from build123d import *

# Parameters (mm, degrees)
SKETCH_W        = 65
SKETCH_H        = 65
PAD_DEPTH       = 16
SKETCH001_W     = 45
SKETCH001_H     = 45
POCKET_DEPTH    = 6
CHAMFER_SIZE    = 13
CHAMFER001_SIZE = 6
CHAMFER002_SIZE = 3


with BuildPart() as part:
    # Sketch → Pad (new body)
    with BuildSketch(Plane.XY):
        with Locations((32.5, 32.5)):
            Rectangle(SKETCH_W, SKETCH_H)
    extrude(amount=PAD_DEPTH)

    # Sketch001 (on Face6 of Pad) → Pocket (cut)
    with BuildSketch(Plane.XY.offset(16)):
        with Locations((32.5, 32.5)):
            Rectangle(SKETCH001_W, SKETCH001_H)
    extrude(amount=-POCKET_DEPTH, mode=Mode.SUBTRACT)

    # Chamfer
    chamfer_edges = [part.edges().sort_by_distance(p)[0] for p in [
        (0, 0, 8),
        (65, 0, 8),
        (65, 65, 8),
        (0, 65, 8),
    ]]
    chamfer(chamfer_edges, length=CHAMFER_SIZE)

    # Chamfer001
    chamfer001_edges = [part.edges().sort_by_distance(p)[0] for p in [
        (32.5, 0, 16),
        (65, 32.5, 16),
        (32.5, 65, 16),
        (0, 32.5, 16),
    ]]
    chamfer(chamfer001_edges, length=CHAMFER001_SIZE)

    # Chamfer002
    chamfer002_edges = [part.edges().sort_by_distance(p)[0] for p in [
        (32.5, 0, 10),
        (65, 32.5, 10),
        (32.5, 65, 10),
        (0, 32.5, 10),
    ]]
    chamfer(chamfer002_edges, length=CHAMFER002_SIZE)


solid = part.part
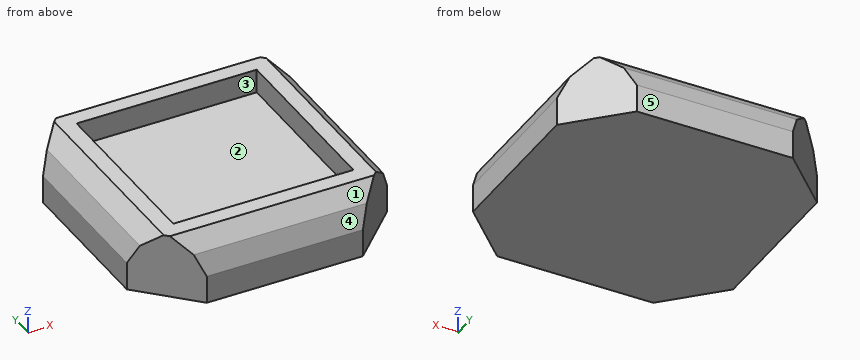
Verification items for the finished model (mm, model axes). Face numbers are marked on the shaded views. A direction names the side the tool comes from. Coordinates: 2 decimals unless noted, no trailing zeros. Order: outer loops, then holes, each group sorted by start corner. A loop starts at its lowest first (then second) coordinate and runs counter-clockwise, first axis right, second up. Notation, with made-up numbers: M 31.25,27 L 37.25,27 A15 cw 37.25,43 Z; hole C -4.75,-38.75 d3. An arc over 180 degrees is marked long. One line per item, written item: value. Start each with the question number.
Item 1: Depth check by flat-ended pin: P1, Ø13.5, axis at x = 34, y = 23.5, coming from the +Z side; P2, Ø1.8, axis at y = 34.5, z = 13, coming from the -X side; P3, Ø4, axis at x = 9, z = 12.5, coming from the +Y side. Enter the tip coordinate at first touch or a pass-through.
Item 2: Sectioned sample at A-A on z = 13.25. Record the cut outline in (x, y), then the cut area to 3 significant figures.
Item 3: Thickness scan on probe 1 along Y at (x, z) = (48, 14.75); probe 2 along Z at (x, y) = (51.5, 29); probe 3 along Y at (x, z) = (15.5, 13.25). Record the ranges inside material, lowest first.
Item 4: Sectioned sample at B-B on y = 17.5. Record the cut outline in (x, z).
Item 5: Access from +Z, -Z, +X, -X, +Y, -Y to the whole of each face (thin tool, end or side, straight path). Record for the marked faces 1 and 2.
Item 6: Sectioned sample at D-D on z = 2.75. Record the cut outline in (x, y).
Item 7: Mould release check, pull along Y, two halves, no side actions. Record for the marked faces 3, 4 and 5: pulls with the +Y half, pulls with the -Y half, needs draft (parallel to the pull), parting line crosses it, or undercut.
Calculated:
1. P1: z = 10
1. P2: x = 2.11
1. P3: y = 62.93
2. outline: M 3.25,9.75 L 9.75,3.25 L 55.25,3.25 L 61.75,9.75 L 61.75,55.25 L 55.25,61.75 L 9.75,61.75 L 3.25,55.25 Z; hole M 10,10 L 55,10 L 55,55 L 10,55 Z
2. area: 1,310 mm^2
3. probe 1: 4.75 to 10, 55 to 60.25
3. probe 2: 0 to 10
3. probe 3: 3.25 to 10, 55 to 61.75
4. outline: M 0,0 L 65,0 L 65,7 L 62.88,12.12 L 59,16 L 55,16 L 55,10 L 10,10 L 10,16 L 6,16 L 2.12,12.12 L 0,7 Z
5. face 1: +Z, +X, -X, -Y
5. face 2: +Z
6. outline: M 0,13 L 13,0 L 52,0 L 65,13 L 65,52 L 52,65 L 13,65 L 0,52 Z
7. face 3: undercut
7. face 4: pulls with the -Y half
7. face 5: pulls with the +Y half
